Verification items for the finished model (mm, model axes). Face numbers are marked on the shaded views. Round coordinates to 2 decimals unless told otherwise and drop trailing zeros. Order: outer loops, then holes, each group sorted by start corner. A loop starts at its lowest first (then second) coordinate and runs counter-clockwise, first axis right, second up. Notation, with made-up numbers: (85, 4) -> (112, 4) arc R19 ccw to (112, 18) -> close; hole circle Ø7 at (-4, 12.5). An arc over 180 degrees is marked (long way). Answer in a Markdown table with one row per item. Add a question column.
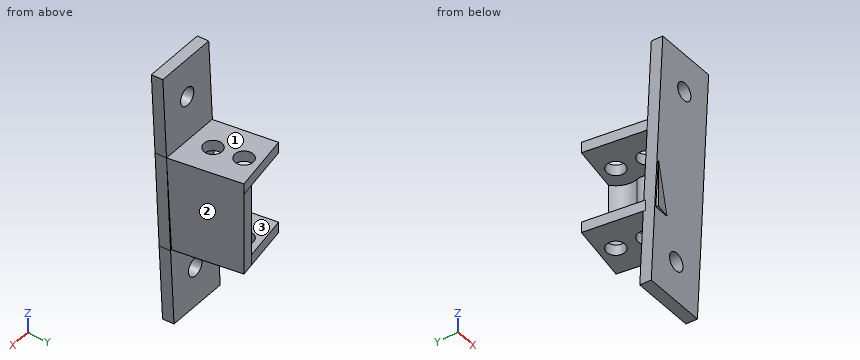
```python
from build123d import *

# Parameters (mm, degrees)
BOSS_EXTRUDE1_DEPTH = 29.21
SKETCH2_R           = 3.175
BOSS_EXTRUDE2_DEPTH = 3.81
BOSS_EXTRUDE3_START = -3.81
SKETCH3_R           = 3.175
BOSS_EXTRUDE3_DEPTH = 3.81
SKETCH4_R           = 3.162370232
SKETCH4_R_2         = 3.091345033
BOSS_EXTRUDE4_DEPTH = 4.064


with BuildPart() as part:
    # Sketch1 → Boss-Extrude1 (new body)
    with BuildSketch(Plane.XY):
        with BuildLine():
            Line((458.862647092, 254.521445295), (448.165127061, 252.766085749))
            Line((448.165127061, 252.766085749), (448.484233443, 250.943633746))
            Line((448.484233443, 250.943633746), (469.389805578, 254.604142486))
            Line((469.389805578, 254.604142486), (465.115245634, 279.016629277))
            Line((465.115245634, 279.016629277), (460.527946701, 278.213405728))
            ThreePointArc((460.527946701, 278.213405728), (463.226929453, 274.636254744), (463.477224231, 270.162121354))
            ThreePointArc((463.477224231, 270.162121354), (463.399405765, 268.135304283), (464.120754615, 266.239598875))
            ThreePointArc((464.120754615, 266.239598875), (464.640877411, 258.967440337), (458.862647092, 254.521445295))
        make_face()
    extrude(amount=-BOSS_EXTRUDE1_DEPTH)

    # Sketch2 → Boss-Extrude2 (add)
    with BuildSketch(Plane.XY):
        Polygon((465.115245634, 279.016629277), (469.389805578, 254.604142486), (448.484233443, 250.943633746), (444.470875732, 275.401856337), align=None)
        with Locations((457.615851502, 262.119672583)):
            Circle(SKETCH2_R, mode=Mode.SUBTRACT)
        with Locations((455.996603091, 271.987703521)):
            Circle(SKETCH2_R, mode=Mode.SUBTRACT)
    extrude(amount=BOSS_EXTRUDE2_DEPTH)

    # Sketch3 → Boss-Extrude3 (add)
    with BuildSketch(Plane(origin=(0, 0, -29.21), x_dir=(-1, 0, 0), z_dir=(0, 0, -1)).offset(BOSS_EXTRUDE3_START)):
        with BuildLine():
            Line((-460.527946701, 278.213405728), (-444.470875732, 275.401856337))
            Line((-444.470875732, 275.401856337), (-448.165127061, 252.766085749))
            Line((-448.165127061, 252.766085749), (-458.862647092, 254.521445295))
            ThreePointArc((-458.862647092, 254.521445295), (-464.640877411, 258.967440337), (-464.120754615, 266.239598875))
            ThreePointArc((-464.120754615, 266.239598875), (-463.399405765, 268.135304283), (-463.477224231, 270.162121354))
            ThreePointArc((-463.477224231, 270.162121354), (-463.226929453, 274.636254744), (-460.527946701, 278.213405728))
        make_face()
        with Locations(Location((-457.615851502, 262.119672583, 0), (0, 0, 180))):
            Circle(SKETCH3_R, mode=Mode.SUBTRACT)
        with Locations(Location((-455.996603091, 271.987703521, 0), (0, 0, 180))):
            Circle(SKETCH3_R, mode=Mode.SUBTRACT)
    extrude(amount=BOSS_EXTRUDE3_DEPTH)

    # Sketch4 → Boss-Extrude4 (add)
    with BuildSketch(Plane(origin=(-3.919475367, 246.715707824, 11.636685294), x_dir=(0.9998741117550616, 0.01584934704377867, 0.0007475562269396132), z_dir=(-0.01586696700779868, 0.9987637706378837, 0.047108065330370395))):
        Polygon((451.768985456, 41.36328589), (451.768985456, 67.563393238), (473.507185402, 67.563393238), (473.507185402, 41.36328589), (473.368872521, 8.189649592), (473.368872521, -19.816380435), (451.768985456, -19.816380435), align=None)
        with Locations(Location((462.696745397, 54.030860165, 0), (0, 0, 270))):
            Circle(SKETCH4_R, mode=Mode.SUBTRACT)
        with Locations(Location((462.696745397, -6.905130234, 0), (0, 0, 270))):
            Circle(SKETCH4_R_2, mode=Mode.SUBTRACT)
    extrude(amount=-BOSS_EXTRUDE4_DEPTH)


solid = part.part
```
1) Cross-section at A-A, the plane y = 273. Record the boundary of the cut face in (x, z) (3 decimals), and give its area (3 significant figures).
2) Cross-section at B-B, the plane x = 447. Record the boundary of the cut face in (y, z), and give its area (3 significant figures).
3) Cross-section at C-C, the plane z = 1.5. Record the boundary of the cut face in (x, y) (3 decimals).
4) Cross-section at D-D, the plane y = 263. Record the boundary of the cut face in (x, z), and give its area (3 significant figures).
5) Thickness scan on L1, parallel to Z at x = 461.5, y = 277; L2, parallel to Y at x = 459.5, z = 3.5; L3, parallel to Z at x = 465.5, y = 269. Record the ranges inside material, lowest first. Write a range as [from, to].
6) Depth check by flat-ended pin: P1, Ø1.5, axis at x = 465.5, z = -36, coming from the -Y side; P2, Ø4, axis at y = 263.5, z = -9.5, coming from the +X side; P3, Ø5, axis at x = 464, z = -43.5, coming from the -Y side. Enter the tip coordinate at first touch or a pass-through.
7) Draft check along Z on the marked faces 1, 2 and 3. Enter one of: +Z half, -Z half, draft (parallel to the pull), parting line (faces both ways), or undercut.
Results below:
| question | item | result |
|---|---|---|
| 1 | outline | (444.863, -29.21) -> (452.987, -29.21) -> (452.987, -25.4) -> (444.863, -25.4) -> close; (444.865, 0) -> (452.987, 0) -> (452.987, 3.81) -> (444.865, 3.81) -> close; (459.006, -29.21) -> (466.169, -29.21) -> (466.169, 3.81) -> (459.006, 3.81) -> (459.006, 0) -> (463.63, 0) -> (463.63, -25.4) -> (459.006, -25.4) -> close |
| 1 | area | 181 mm² |
| 2 | outline | (259.91, -29.21) -> (275.84, -29.21) -> (275.84, -25.4) -> (259.91, -25.4) -> close; (259.99, 0) -> (275.84, 0) -> (275.84, 3.81) -> (259.99, 3.81) -> close |
| 2 | area | 121 mm² |
| 3 | outline | (444.471, 275.402) -> (447.922, 254.372) -> (447.793, 254.37) -> (447.857, 250.302) -> (469.463, 250.645) -> (469.399, 254.713) -> (469.371, 254.713) -> (465.115, 279.017) -> close; hole circle Ø6.35 at (455.997, 271.988); hole circle Ø6.35 at (457.616, 262.12) |
| 4 | outline | (446.49, -29.21) -> (454.57, -29.21) -> (454.57, -25.4) -> (446.49, -25.4) -> close; (446.51, 0) -> (454.57, 0) -> (454.57, 3.81) -> (446.51, 3.81) -> close; (460.67, -29.21) -> (467.92, -29.21) -> (467.92, 3.81) -> (460.67, 3.81) -> (460.67, 0) -> (465.27, 0) -> (465.27, -25.4) -> (460.67, -25.4) -> close |
| 4 | area | 184 mm² |
| 5 | L1 | [-29.21, -25.4], [0, 3.81] |
| 5 | L2 | [250.39, 259.56], [264.68, 278.03] |
| 5 | L3 | [-29.21, 3.81] |
| 6 | P1 | y = 252.31 |
| 6 | P2 | x = 468.18 |
| 6 | P3 | y = 252.56 |
| 7 | face 1 | +Z half |
| 7 | face 2 | draft |
| 7 | face 3 | undercut |
